```python
from build123d import *

# Parameters (mm, degrees)
BOSS_EXTRUDE1_START     = -2.5
SKETCH1_W               = 70
SKETCH1_H               = 39.95
BOSS_EXTRUDE1_DEPTH     = 2.5
SKETCH2_W               = 60
SKETCH2_H               = 2.6
BOSS_EXTRUDE2_DEPTH     = 13.5
SKETCH3_W               = 60
SKETCH3_H               = 2.6
BOSS_EXTRUDE3_DEPTH     = 13.5
SKETCH4_R               = 2.75
BOSS_EXTRUDE4_DEPTH     = 13.5
BOSS_EXTRUDE5_START     = -19
SKETCH5_R               = 5
BOSS_EXTRUDE5_DEPTH     = 16.5
CUT_EXTRUDE1_DEPTH      = 46.343143087
CUT_EXTRUDE1_DEPTH_BACK = 46.343143087
SKETCH6_W               = 22.8
SKETCH6_H               = 11.9
CUT_EXTRUDE2_DEPTH      = 46.343143087
CUT_EXTRUDE2_DEPTH_BACK = 46.343143087
SKETCH7_R               = 0.9
CUT_EXTRUDE3_DEPTH      = 46.343143087
CUT_EXTRUDE3_DEPTH_BACK = 46.343143087
SKETCH8_R               = 0.9
CUT_EXTRUDE4_DEPTH      = 46.343143087
CUT_EXTRUDE4_DEPTH_BACK = 46.343143087
SKETCH9_R               = 1.725
CUT_EXTRUDE5_START      = -4.2
CUT_EXTRUDE5_DEPTH      = 4.2


with BuildPart() as part:
    # Sketch1 → Boss-Extrude1 (new body)
    with BuildSketch(Plane.XY.offset(BOSS_EXTRUDE1_START)):
        Rectangle(SKETCH1_W, SKETCH1_H)
    extrude(amount=BOSS_EXTRUDE1_DEPTH)

    # Sketch2 → Boss-Extrude2 (add)
    with BuildSketch(Plane.XY):
        with Locations((-5, 16.975)):
            Rectangle(SKETCH2_W, SKETCH2_H)
    extrude(amount=BOSS_EXTRUDE2_DEPTH)

    # Sketch3 → Boss-Extrude3 (add)
    with BuildSketch(Plane.XY):
        with Locations((5, -16.975)):
            Rectangle(SKETCH3_W, SKETCH3_H)
    extrude(amount=BOSS_EXTRUDE3_DEPTH)

    # Sketch4 → Boss-Extrude4 (add)
    with BuildSketch(Plane.XY):
        with Locations((-8, 16.975)):
            Circle(SKETCH4_R)
        with Locations((8, -16.975)):
            Circle(SKETCH4_R)
    extrude(amount=BOSS_EXTRUDE4_DEPTH)

    # Sketch5 → Boss-Extrude5 (add)
    with BuildSketch(Plane.XY.offset(BOSS_EXTRUDE5_START)):
        with Locations(Location((-31, 6, 0), (0, 0, 143.130102354))):
            Circle(SKETCH5_R)
        with Locations(Location((-31, -6, 0), (0, 0, 143.130102354))):
            Circle(SKETCH5_R)
    extrude(amount=BOSS_EXTRUDE5_DEPTH)

    # Sketch6 → Cut-Extrude1 (cut, two sides: drawn at the far end of the back side and taken through both)
    with BuildSketch(Plane.XY.offset(-CUT_EXTRUDE1_DEPTH_BACK)):
        with Locations((5.8, 0)):
            Rectangle(SKETCH6_W, SKETCH6_H)
    extrude(amount=CUT_EXTRUDE1_DEPTH + CUT_EXTRUDE1_DEPTH_BACK, mode=Mode.SUBTRACT)

    # Sketch7 → Cut-Extrude2 (cut, two sides: drawn at the far end of the back side and taken through both)
    with BuildSketch(Plane.XY.offset(-CUT_EXTRUDE2_DEPTH_BACK)):
        with Locations((-7.95, 0)):
            Circle(SKETCH7_R)
        with Locations((19.55, 0)):
            Circle(SKETCH7_R)
    extrude(amount=CUT_EXTRUDE2_DEPTH + CUT_EXTRUDE2_DEPTH_BACK, mode=Mode.SUBTRACT)

    # Sketch8 → Cut-Extrude3 (cut, two sides: drawn at the far end of the back side and taken through both)
    with BuildSketch(Plane.XY.offset(-CUT_EXTRUDE3_DEPTH_BACK)):
        with Locations((-8, 16.975)):
            Circle(SKETCH8_R)
        with Locations((8, -16.975)):
            Circle(SKETCH8_R)
    extrude(amount=CUT_EXTRUDE3_DEPTH + CUT_EXTRUDE3_DEPTH_BACK, mode=Mode.SUBTRACT)

    # Sketch9 → Cut-Extrude4 (cut, two sides: drawn at the far end of the back side and taken through both)
    with BuildSketch(Plane.XY.offset(-CUT_EXTRUDE4_DEPTH_BACK)):
        with Locations((-31, 6)):
            Circle(SKETCH9_R)
        with Locations((-31, -6)):
            Circle(SKETCH9_R)
    extrude(amount=CUT_EXTRUDE4_DEPTH + CUT_EXTRUDE4_DEPTH_BACK, mode=Mode.SUBTRACT)

    # Sketch10 → Cut-Extrude5 (cut)
    with BuildSketch(Plane.XY.offset(CUT_EXTRUDE5_START)):
        Polygon((-28.2, 7.616580754), (-31, 9.233161507), (-33.8, 7.616580754), (-33.8, 4.383419246), (-31, 2.766838493), (-28.2, 4.383419246), align=None)
        Polygon((-28.2, -4.383419246), (-31, -2.766838493), (-33.8, -4.383419246), (-33.8, -7.616580754), (-31, -9.233161507), (-28.2, -7.616580754), align=None)
    extrude(amount=CUT_EXTRUDE5_DEPTH, mode=Mode.SUBTRACT)


solid = part.part
```
Build history of the part. All positions in model axes, mm. A direction names the side the tool comes from. Coordinates: 2 decimals unless noted, no trailing zeros. Order: outer loops, then holes, each group sorted by start corner. A loop starts at its lowest first (then second) coordinate and runs counter-clockwise, first axis right, second up. Notation, with made-up numbers: (10.5, -14) -> (20.5, -14) arc R24 ccw to (20.5, 1) -> close; hole circle Ø8 at (69, 8.5). An arc over 180 degrees is marked (long way). Answer in a Markdown table with one row per item. Add a question column.
Q1. Band-saw the part on A-A, the plane x = 19.55. List the corners of the cut face in (y, z) (3 decimals), then the cut area to 3 significant figures.
Q2. Band-saw the part on C-C, the plane z = 11. List the corners of the cut face in (x, y) (3 decimals).
Q3. Drop flat-ended pins along their axis: pin 1 (6 mm diameter, centred on y = -9.5, z = 1.5, fed in from -X); pin 2 (8 mm diameter, centred on x = -7.5, y = 9, fed in from +Z); pin 3 (4 mm diameter, centred on y = 10, z = -5, fed in from -X). Give the stop position or say it passes through.
Q4. Wall check: line 1 along X through (y, z) = (0, -1.9); line 2 along Y through (x, z) = (-31, -8.25) (3 decimals); line 3 along Y through (x, z) = (-14.5, 12.5) (3 decimals). Give the ranges that are in metal, low to high. Write a range as [from, to].
Q5. Which spindle directions (+Z, -Z, +X, -X, +Y, -Y) get a long thin tool onto all of the face, cutting with end or side? Do faces 1 (the face through (6, 5.95, -1)), 2 (the face through (-28.2, 6, -2)), 3 (the face through (-23, 15.675, 7)), 4 (the face through (23, -18.275, 7)), 5 (the face through (-35.716, 7.66, -10.866)). Say none if no direction does.
Q6. Band-saw the part on B-B, the plane y = 0. List the corners of the cut face in (x, z), then the cut area to 3 significant figures.
Q7. Band-saw the part on D-D, the plane z = -1.5. List the corners of the cut face in (x, y) (3 decimals), then the cut area to 3 significant figures.
Q8. Mould opens along Y. For faces 6 (the face through (-25, -17, 7)), 7 (the face through (-7.958, 19.725, 6.656)), 8 (the face through (17.2, 0, -1)) say: +Y half, -Y half, draft (parallel to the pull), parting line (faces both ways), or undercut.
Answers follow:
| question | item | result |
|---|---|---|
| 1 | outline | (-19.975, -2.5) -> (-0.9, -2.5) -> (-0.9, 0) -> (-15.675, 0) -> (-15.675, 13.5) -> (-18.275, 13.5) -> (-18.275, 0) -> (-19.975, 0) -> close; (0.9, -2.5) -> (19.975, -2.5) -> (19.975, 0) -> (18.275, 0) -> (18.275, 13.5) -> (15.675, 13.5) -> (15.675, 0) -> (0.9, 0) -> close |
| 1 | area | 166 mm^2 |
| 2 | outline | (-35, 15.675) -> (-10.423, 15.675) arc R2.75 ccw to (-5.577, 15.675) -> (25, 15.675) -> (25, 18.275) -> (-5.577, 18.275) arc R2.75 ccw to (-10.423, 18.275) -> (-35, 18.275) -> close; (-25, -18.275) -> (5.577, -18.275) arc R2.75 ccw to (10.423, -18.275) -> (35, -18.275) -> (35, -15.675) -> (10.423, -15.675) arc R2.75 ccw to (5.577, -15.675) -> (-25, -15.675) -> close; hole circle Ø1.8 at (-8, 16.975); hole circle Ø1.8 at (8, -16.975) |
| 3 | pin 1 | x = -35 |
| 3 | pin 2 | z = 0 |
| 3 | pin 3 | x = -35.58 |
| 4 | line 1 | [-35, -8.85], [-7.05, -5.6], [17.2, 18.65], [20.45, 35] |
| 4 | line 2 | [-11, -7.725], [-4.275, -1], [1, 4.275], [7.725, 11] |
| 4 | line 3 | [-18.275, -15.675], [15.675, 18.275] |
| 5 | face 1 | +Z, -Z |
| 5 | face 2 | +Z |
| 5 | face 3 | +Z, -X |
| 5 | face 4 | +Z, +X, -Y |
| 5 | face 5 | -Z |
| 6 | outline | (-35, -2.5) -> (-8.85, -2.5) -> (-8.85, 0) -> (-35, 0) -> close; (-7.05, -2.5) -> (-5.6, -2.5) -> (-5.6, 0) -> (-7.05, 0) -> close; (17.2, -2.5) -> (18.65, -2.5) -> (18.65, 0) -> (17.2, 0) -> close; (20.45, -2.5) -> (35, -2.5) -> (35, 0) -> (20.45, 0) -> close |
| 6 | area | 109 mm^2 |
| 7 | outline | (-35, -19.975) -> (35, -19.975) -> (35, 19.975) -> (-35, 19.975) -> close; hole (-33.8, -7.617) -> (-31, -9.233) -> (-28.2, -7.617) -> (-28.2, -4.383) -> (-31, -2.767) -> (-33.8, -4.383) -> close; hole (-33.8, 4.383) -> (-31, 2.767) -> (-28.2, 4.383) -> (-28.2, 7.617) -> (-31, 9.233) -> (-33.8, 7.617) -> close; hole circle Ø1.8 at (-8, 16.975); hole circle Ø1.8 at (-7.95, 0); hole (-5.6, -5.95) -> (17.2, -5.95) -> (17.2, 5.95) -> (-5.6, 5.95) -> close; hole circle Ø1.8 at (8, -16.975); hole circle Ø1.8 at (19.55, 0) |
| 7 | area | 2,460 mm^2 |
| 8 | face 6 | draft |
| 8 | face 7 | +Y half |
| 8 | face 8 | undercut |
